Autodesk Inventor part; units mm, degrees
ref_plane "YZ Plane" through (0, 0, 0) normal (1, 0, 0) x (0, 1, 0)
ref_plane "XZ Plane" through (0, 0, 0) normal (0, 1, 0) x (-1, 0, 0)
ref_plane "XY Plane" through (0, 0, 0) normal (0, 0, 1) x (1, 0, 0)
sketch "Эскиз1" plane through (0, 0, 0) normal (0, 0, 1) x (1, 0, 0)
  line L0 (-63.5, -92.5) -> (-63.5, -81)
  line L1 (-63.5, -81) -> (-63.5, -92.5)
  line L2 (-75.5, -92.5) -> (-75.5, -80.5)
  line L3 (-97.5, -62.5) -> (-68.5, -62.5)
  line L4 (-68.5, -62.5) -> (-68.5, -52.5)
  line L5 (-68.5, -52.5) -> (-63.5, -52.5)
  line L6 (-63.5, -52.5) -> (-63.5, -76)
  line L7 (-63.5, -76) -> (-53.5, -76)
  line L8 (-53.5, -76) -> (-53.5, -81)
  line L9 (-63.5, -92.5) -> (-75.5, -92.5)
  line L10 (-53.5, -81) -> (-63.5, -81)
  line L11 (-97.5, -70) -> (-91.5, -70)
  line L12 (-91.5, -70) -> (-75.5, -80.5)
  line L13 (-97.5, -62.5) -> (-97.5, -70)
  line L14 (-117, 0) -> (19.5, 0)
  point P0 (0, 0)
  dimension "d0" = 12
  dimension "d1" = 5
  dimension "d2" = 10
  dimension "d3" = 30
  dimension "d5" = 12
  dimension "d7" = 10
  dimension "d8" = 6
  dimension "d9" = 5
  dimension "d10" = 7.5
  dimension "d11" = 22
  dimension "d13" = 70
revolve "Вращение1" add sketch "Эскиз1" angle 360 about axis through (-10, 0, 0) along (1, 0, 0)
chamfer "Фаска1" distance 2 angle 45 1 edges at (-97.5, 70, 0)
chamfer "Фаска2" distance 2 angle 45 1 edges at (-97.5, 62.5, 0)
chamfer "Фаска3" distance 2 angle 45 1 edges at (-53.5, 81, 0)
hole "Отверстие2" at (-75.5, -86.0624, 0.0573) direction (1, 0, 0) diameter 6 end through all counterbore diameter 9 counterbore depth 5
pattern_circular "Круговой массив2" count 6 over 360 about axis through (-10, 0, 0) along (1, 0, 0) of "Отверстие2"
properties part number "2 крышка"
Geometry check sheet. Reference: the model listing, model coordinates, mm. A direction names the side the tool comes from. Round coordinates to 2 decimals unless told otherwise and drop trailing zeros. Loops run counter-clockwise (first coordinate to the right, second up) from the corner with the lowest first, then second, coordinate; pieces in that order, holes last. Notation, with made-up numbers: (51, 41.25) -> (96, 41.25) arc R20 ccw to (96, 62.25) -> close; hole circle Ø5 at (42, 51). An arc over 180 degrees is marked (long way). Answer as a JSON object with one key per item and string values. Group by question number.
Item 1: Release check for a two-part mould opening along Z. For faces 4 (the face through (-66.951, 89.037, 0.333)), 5 (the face through (-97.375, -64.979, -20.463)), 6 (the face through (-75.5, 76, -28)) record: pulls with the +Z half, pulls with the -Z half, needs draft (parallel to the pull), parting line crosses it, or undercut.
Item 2: Set-up check for faces 1 (the face through (-70.5, 83, -1)), 2 (the face through (-66.95, 44.13, -71.79)), 3 (the face through (-63.5, 18, 50)): record each of +Z, -Z, +X, -X, +Y, -Y from which the full face is reachable in a straight line by a thin tool's end or side.
Item 3: Depth check by flat-ended pin: pin 1 Ø10 at (x, y) = (-89, -68.5) entering from +Z; pin 2 Ø7 at (y, z) = (-41.5, 75) entering from -X; pin 3 Ø12 at (x, z) = (-70.5, -9) entering from -Y; pin 4 Ø5 at (y, z) = (7.5, -47.5) entering from +X. Enter the tip coordinate at first touch or a pass-through.
Item 4: Cross-section at B-B, the plane x = -59.5. Record the cut outline in (y, z), plus the area to 3 significant figures.
Item 5: Cross-section at C-C, the plane z = 0. Count the separate pieces of the cut face and the enclosed holes in it, plus the area to 3 significant figures.
Item 6: Thickness scan on line 1 along Y through (x, z) = (-65, 0); line 2 along Z through (x, y) = (-58.5, -1); line 3 along Z through (x, y) = (-72, -45). Record the ranges inside material, lowest first.
Determined:
{
 "1": {"face 4": "undercut", "face 5": "parting line crosses it", "face 6": "needs draft"},
 "2": {"face 1": "-X", "face 2": "+X, -X", "face 3": "+X"},
 "3": {"pin 1": "stops at z = 35.47", "pin 2": "stops at x = -75.5", "pin 3": "stops at y = -92.45", "pin 4": "passes through"},
 "4": {"outline": "circle Ø162 at (0, 0); hole circle Ø152 at (0, 0)", "area": "2,470 mm²"},
 "5": {"separate pieces": "4", "enclosed holes": "0", "area": "1,230 mm²"},
 "6": {"line 1": "y = -92.5 to -89.06, -83.06 to -52.5, 52.5 to 83.06, 89.06 to 92.5", "line 2": "z = -80.99 to -75.99, 75.99 to 80.99", "line 3": "z = -80.82 to -78.57, -70.43 to -43.37, 43.37 to 70.54, 78.58 to 80.82"}
}
